Study the drawing (mm; zero at the part's minimum x, y, z) and answer. Coordinates: 2 decimals unless noted, no trailing zeros. Loops run counter-clockwise (first coordinate to the right, second up) from the corner with the lowest first, then second, coordinate; pieces in that order, holes last. Notation, with made-up numbers: (-18, 42.25) - (37, 42.25) arc R25 cw to (37, 64.25) - close; hole circle Ø11 at (-4.75, -19). An arc over 180 degrees is marked (long way). Write each question's results on one line, items separated by ' | '. Start each with the question number.
(1) Given pin 1 Ø24 at (y, z) = (60, 57.5) entering from +X; pin 2 Ø12 at (x, z) = (39.5, 36.5) entering from +Y; pin 3 Ø5 at (y, z) = (131.5, 57) entering from +X, each flat-ended and moving along its own axis, determine where each tip first touches the part or whether it passes through.
(2) Find section A-A on z = 57.5. Determine the outline of the cut face in (x, y).
(3) Find section D-D on y = 130. Determine the outline of the cut face in (x, z).
(4) Find section B-B on x = 32.5. Determine the outline of the cut face in (y, z), then the cut area to 3 significant figures.
(5) Find section C-C on y = 60. Determine the outline of the cut face in (x, z), then the cut area to 3 significant figures.
(6) Consider line 1 (Y direction, x = 7, z = 57); line 2 (X direction, y = 45, z = 91). Determine where each line is inside the solid, lowest interval first. Write a range as from..to.
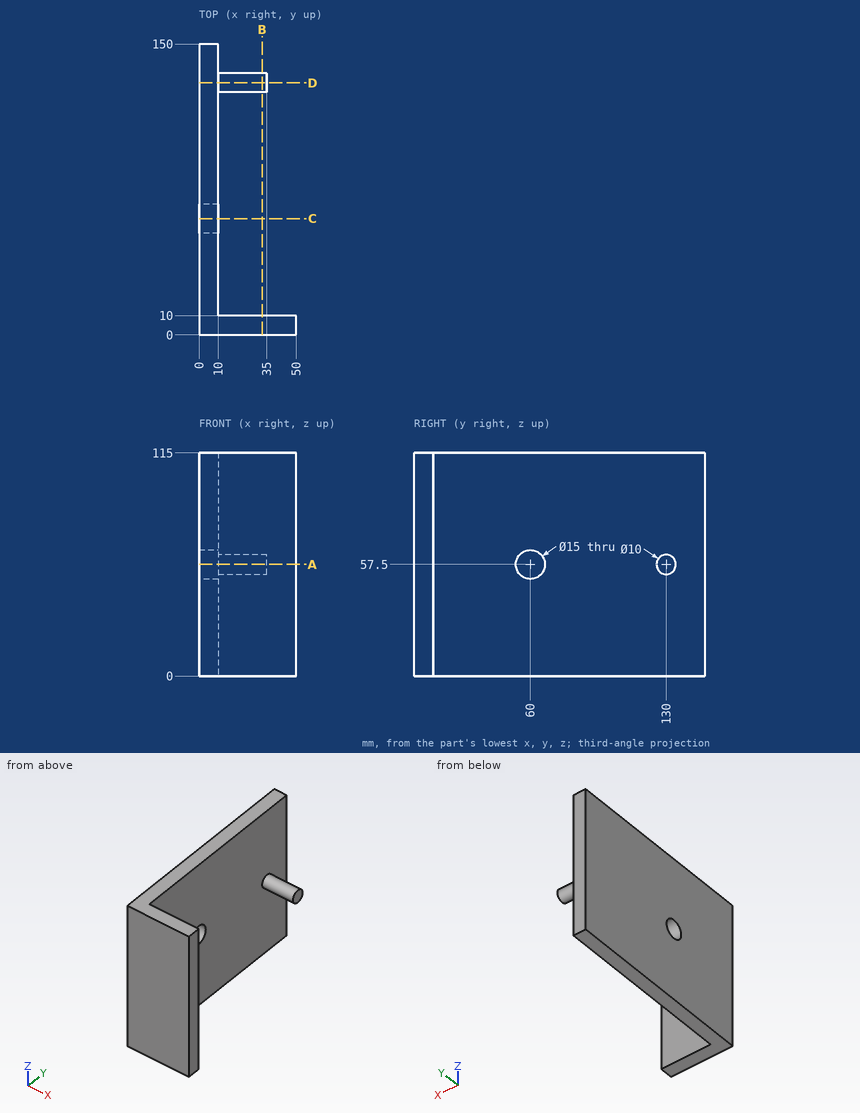
Values:
1) pin 1: stops at x = 10 | pin 2: stops at y = 10 | pin 3: stops at x = 35
2) outline: (0, 0) - (50, 0) - (50, 10) - (10, 10) - (10, 52.5) - (0, 52.5) - close; (0, 67.5) - (10, 67.5) - (10, 125) - (35, 125) - (35, 135) - (10, 135) - (10, 150) - (0, 150) - close
3) outline: (0, 0) - (10, 0) - (10, 52.5) - (35, 52.5) - (35, 62.5) - (10, 62.5) - (10, 115) - (0, 115) - close
4) outline: (0, 0) - (10, 0) - (10, 115) - (0, 115) - close; circle Ø10 at (130, 57.5) | area: 1,230 mm²
5) outline: (0, 0) - (10, 0) - (10, 50) - (0, 50) - close; (0, 65) - (10, 65) - (10, 115) - (0, 115) - close | area: 1,000 mm²
6) line 1: y = 0..52.52, 67.48..150 | line 2: x = 0..10
